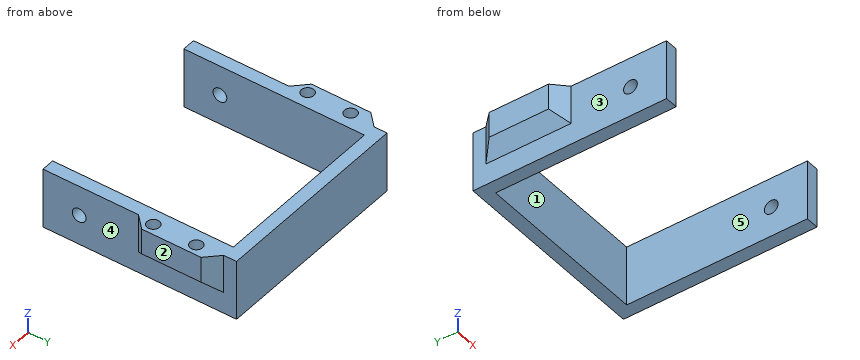
```python
from build123d import *

# Parameters (mm, degrees)
F1_DEPTH = 14
F2_W     = 6
F2_H     = 19.8
F3_DEPTH = 9
F4_R     = 1.45
F5_DEPTH = 6.5
F6_SIZE  = 2.99999
F7_R     = 1.6
F8_DEPTH = 3
F10_SIZE = 1.45


# Not quite as in the source:
# - a fillet or chamfer is up to 0.001 mm smaller than in the source, because OpenCascade refuses the exact size


with BuildPart() as f1:
    # F0 (on Top) → F1 (new body)
    with BuildSketch(Plane.XY):
        Polygon((0, 24.2671520197), (0, 21.2671520197), (20.4, 21.2671520197), (20.4, -20.7328479803), (23.4, -20.7328479803), (23.4, 24.2671520197), align=None)
    extrude(amount=F1_DEPTH)

    # F2 (on face) → F3 (join)
    with BuildSketch(Plane.XY.offset(14)):
        with Locations((23.4, 11.3671520197)):
            Rectangle(F2_W, F2_H)
    extrude(amount=-F3_DEPTH)

    # F4 (on face) → F5 (cut)
    with BuildSketch(Plane.XY.offset(14)):
        with Locations((24, 5.3671520197)):
            Circle(F4_R)
        with Locations((24, 15.3671520197)):
            Circle(F4_R)
    extrude(amount=-F5_DEPTH, mode=Mode.SUBTRACT)

    # F6 (size 3 in the source; OpenCascade refuses exactly that, so slightly less here)
    f6_edges = [f1.edges().sort_by_distance(p)[0] for p in [
        (26.4, 1.467152, 9.5),
        (26.4, 21.267152, 9.5),
        (26.4, 11.367152, 5),
    ]]
    chamfer(f6_edges, length=F6_SIZE)

    # F7 (on face) → F8 (cut, through all)
    with BuildSketch(Plane.YZ.offset(23.4)):
        with Locations((-12.3328479803, 7)):
            Circle(F7_R)
    extrude(amount=-F8_DEPTH, mode=Mode.SUBTRACT)

    # F9: F1 across plane


with BuildPart() as f1_1:
    add(f1.part)
    add(f1.part.mirror(Plane.YZ))

    # F10
    f10_edges = [f1_1.edges().sort_by_distance(p)[0] for p in [
        (22.55, 15.367152, 7.5),
        (22.55, 5.367152, 7.5),
        (-22.55, 5.367152, 7.5),
        (-22.55, 15.367152, 7.5),
    ]]
    chamfer(f10_edges, length=F10_SIZE)


solid = f1_1.part
```
Input: part model. Units: mm. Frame: model coordinates. Face numbers are marked on the shaded views. A direction names the side the tool comes from. Coordinates: 2 decimals unless noted, no trailing zeros. Write each loop counter-clockwise with the first axis right and the second up, starting at its lowest first coordinate (ties: lowest second). Pieces come first, ordered by that corner, then holes.
1) Pin query (flat end, axial travel): pin 1 Ø3.5 at (y, z) = (-12.33, 7) entering from -X; pin 2 Ø7 at (y, z) = (-5, 10.5) entering from +X; pin 3 Ø2.5 at (x, y) = (24, 5.37) entering from +Z. Return the tip coordinate at first contact, or that it passes through.
2) Section C-C on z = 2. Output: boundary loops of the cut face in (x, y), and give its area (3 significant figures).
3) Material intervals for line 1 along X through (y, z) = (1, 1.25); line 2 along Y through (x, z) = (24, 11.45); line 3 along Y through (x, z) = (-2, 13.25), sorted ascending.
4) Section A-A on y = -8. Output: boundary loops of the cut face in (x, z), and give its area (3 significant figures).
5) Section B-B on z = 6.25. State how many separate pieces and enclosed holes the cut face has, and give its area (3 significant figures).
6) Set-up query: the marked faces 1 and 2. Return all of +Z, -Z, +X, -X, +Y, -Y with unobstructed straight access to the full face (end or side cutting, diameter ignored); none if empty.
7) Mould query, pull axis X, two halves, no side actions, for the marked faces 3, 4 and 5. Classes: pulls with the +X half, pulls with the -X half, needs draft (parallel to the pull), parting line crosses it, or undercut.
Check result:
1. pin 1: stops at x = -23.4
1. pin 2: stops at x = 23.4
1. pin 3: stops at z = 8.75
2. outline: (-23.4, -20.73) - (-20.4, -20.73) - (-20.4, 21.27) - (20.4, 21.27) - (20.4, -20.73) - (23.4, -20.73) - (23.4, 24.27) - (-23.4, 24.27) - close
2. area: 392 mm2
3. line 1: x = -23.4 to -20.4, 20.4 to 23.4
3. line 2: y = 2.07 to 3.92, 6.82 to 13.92, 16.82 to 20.67
3. line 3: y = 21.27 to 24.27
4. outline: (-23.4, 0) - (-20.4, 0) - (-20.4, 14) - (-23.4, 14) - close; (20.4, 0) - (23.4, 0) - (23.4, 14) - (20.4, 14) - close
4. area: 84.0 mm2
5. separate pieces: 3
5. enclosed holes: 0
5. area: 422 mm2
6. face 1: +Z, -Z, -Y
6. face 2: +Z, -Z, +X, +Y, -Y
7. face 3: pulls with the -X half
7. face 4: pulls with the +X half
7. face 5: undercut
